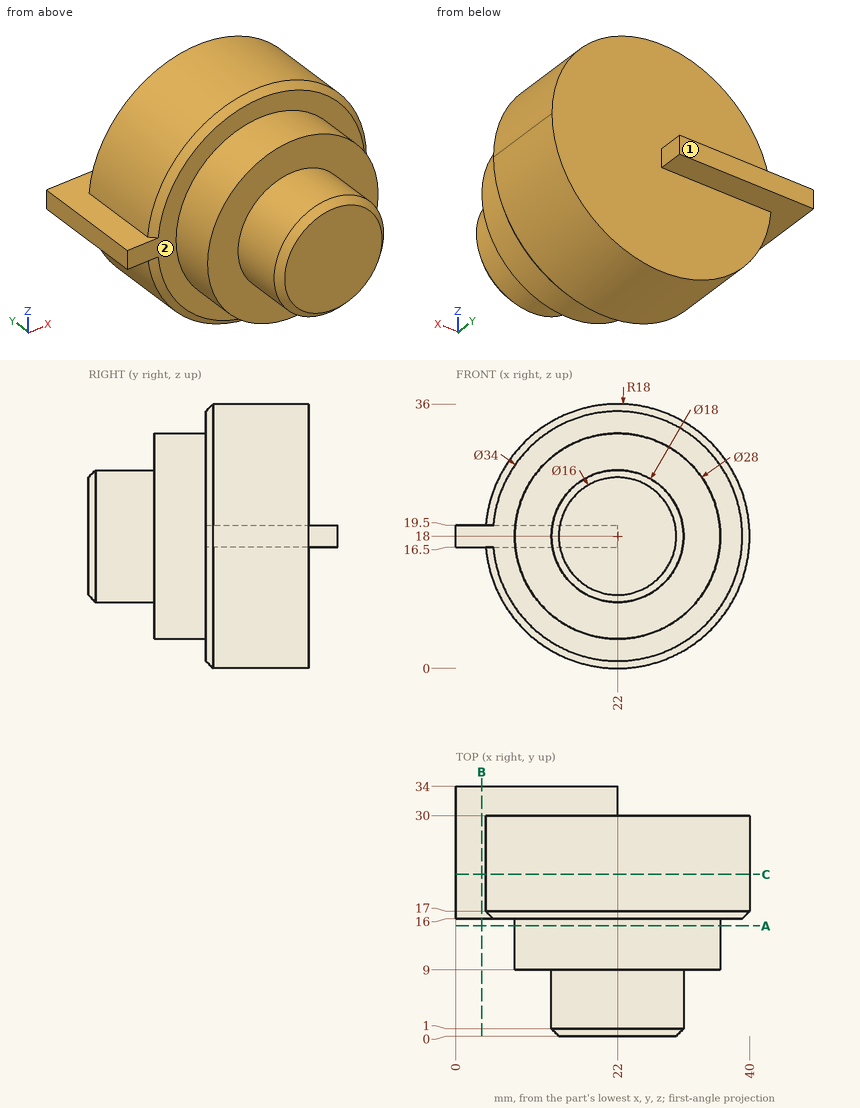
Drawing for the job (mm, zero at the part's lowest x, y, z). A direction names the side the tool comes from. Give positions to 0.01 mm unless a question says otherwise; leave off trailing zeros. Order: outer loops, then holes, each group sorted by start corner. A loop starts at its lowest first (then second) coordinate and runs counter-clockwise, first axis right, second up. Notation, with made-up numbers: M 74,-8 L 132,-8 A13 ccw 132,17 Z; hole C 49,59.25 d4. An arc over 180 degrees is marked long. Put each result on its own line as item: value.
Item 1: 3-axis set-ups, long thin cutter, end or side, ignore diameter. For the marked faces 1 and 2: which of +Z, -Z, +X, -X, +Y, -Y reach the whole face in a straight line?
From the geometry:
face 1: +Z, -Z, +X, -X, +Y
face 2: -Y
Item 2: Slice it at A-A, the plane y = 15. Write the cut outline in (x, z).
From the geometry:
outline: C 22,18 d28
Item 3: Slice it at C-C, the plane y = 22. Write the cut outline in (x, z).
From the geometry:
outline: M 0,16.5 L 4.06,16.5 A18 ccw long 4.06,19.5 L 0,19.5 Z
Item 4: Slice it at B-B, the plane x = 3.5. Write the cut outline in (y, z).
From the geometry:
outline: M 16,16.5 L 34,16.5 L 34,19.5 L 16,19.5 Z
Item 5: Flat gauge pins, fed straight in: pin 1 Ø6 at (x, z) = (5, 21.5) entering from -Y; pin 2 Ø12 at (y, z) = (23, 9) entering from -X; pin 3 Ø8 at (y, z) = (6.5, 31.5) entering from +X; pin 4 Ø5 at (x, y) = (4.5, 13) entering from +Z. Where does each tip first touch, or does it go through?
From the geometry:
pin 1: stops at y = 16
pin 2: stops at x = 4.25
pin 3: stops at x = 31.4
pin 4: passes through
Item 6: Probe line 1 (Z direction, x = 6, y = 30.5); line 2 (Y direction, x = 7, z = 19); line 3 (Y direction, x = 27.5, z = 18.5). List the from-to ranges inside material, lowest first. Write a range as [from, to].
From the geometry:
line 1: z = [16.5, 19.5]
line 2: y = [16, 34]
line 3: y = [0, 30]
